```python
from build123d import *

# Parameters (mm, degrees)
SKETCH_1_W           = 76.35
SKETCH_1_H           = 54
EXTRUDE_7_DEPTH      = 5
EXTRUDE_7_DEPTH_BACK = 5
EXTRUDE_8_DEPTH      = 12.5
EXTRUDE_8_DEPTH_BACK = 80
SKETCH_3_W           = 4.5
SKETCH_3_H           = 4
SKETCH_3_W_2         = 4
SKETCH_3_H_2         = 40.6
EXTRUDE_9_DEPTH      = 12.5
SKETCH_5_R           = 1.25
CUT_EXTRUDE_1_DEPTH  = 12.5
FILLET_1_R           = 4
FILLET_2_R           = 4
FILLET_3_R           = 8
FILLET_4_R           = 8
FILLET_5_R           = 8
FILLET_6_R           = 8
FILLET_7_R           = 5
FILLET_8_R           = 5
FILLET_9_R           = 4
FILLET_10_R          = 4


with BuildPart() as part:
    # Sketch 1 → Extrude 7 (new body, two sides)
    with BuildSketch(Plane.XY) as extrude_7_sk:
        with Locations((38.175, -23)):
            Rectangle(SKETCH_1_W, SKETCH_1_H)
        Polygon((4, -46), (4, -39), (9, -39), (9, -36.6), (4, -36.6), (4, 0), (72.35, 0), (72.35, -36.6), (67.35, -36.6), (67.35, -39), (72.35, -39), (72.35, -46), align=None, mode=Mode.SUBTRACT)
    extrude(amount=EXTRUDE_7_DEPTH)
    extrude(extrude_7_sk.sketch, amount=-EXTRUDE_7_DEPTH_BACK)

    # Sketch 2 → Extrude 8 (add, two sides)
    with BuildSketch(Plane.XY.offset(5)) as extrude_8_sk:
        Polygon((4, -46), (4, -39), (9, -39), (9, -36.6), (4, -36.6), (0, -36.6), (0, -50), (76.35, -50), (76.35, -36.6), (72.35, -36.6), (67.35, -36.6), (67.35, -39), (72.35, -39), (72.35, -46), align=None)
    extrude(amount=EXTRUDE_8_DEPTH)
    extrude(extrude_8_sk.sketch, amount=-EXTRUDE_8_DEPTH_BACK)

    # Sketch 3 → Extrude 9 (add)
    with BuildSketch(Plane.XY.offset(5)):
        with Locations((52.065, 2)):
            Rectangle(SKETCH_3_W, SKETCH_3_H)
        with Locations((24.285, 2)):
            Rectangle(SKETCH_3_W, SKETCH_3_H)
        with Locations((2, -16.3)):
            Rectangle(SKETCH_3_W_2, SKETCH_3_H_2)
        with Locations((74.35, -16.3)):
            Rectangle(SKETCH_3_W_2, SKETCH_3_H_2)
    extrude(amount=EXTRUDE_9_DEPTH)

    # Sketch 5 → Cut-Extrude 1 (cut)
    with BuildSketch(Plane(origin=(0, 4, 0), x_dir=(1, 0, 0), z_dir=(0, 1, 0))):
        with Locations((24.285, -12.5)):
            Circle(SKETCH_5_R)
        with Locations((52.065, -12.5)):
            Circle(SKETCH_5_R)
    extrude(amount=-CUT_EXTRUDE_1_DEPTH, mode=Mode.SUBTRACT)

    # Fillet 1
    fillet_1_edges = [part.edges().sort_by_distance(p)[0] for p in [
        (2, -36.6, -5),
    ]]
    fillet(fillet_1_edges, radius=FILLET_1_R)

    # Fillet 2
    fillet_2_edges = [part.edges().sort_by_distance(p)[0] for p in [
        (74.35, -36.6, -5),
    ]]
    fillet(fillet_2_edges, radius=FILLET_2_R)

    # Fillet 3
    fillet_3_edges = [part.edges().sort_by_distance(p)[0] for p in [
        (4, 2, 5),
    ]]
    fillet(fillet_3_edges, radius=FILLET_3_R)

    # Fillet 4
    fillet_4_edges = [part.edges().sort_by_distance(p)[0] for p in [
        (72.35, 2, 5),
    ]]
    fillet(fillet_4_edges, radius=FILLET_4_R)

    # Fillet 5
    fillet_5_edges = [part.edges().sort_by_distance(p)[0] for p in [
        (22.035, 2, 5),
    ]]
    fillet(fillet_5_edges, radius=FILLET_5_R)

    # Fillet 6
    fillet_6_edges = [part.edges().sort_by_distance(p)[0] for p in [
        (54.315, 2, 5),
    ]]
    fillet(fillet_6_edges, radius=FILLET_6_R)

    # Fillet 7
    fillet_7_edges = [part.edges().sort_by_distance(p)[0] for p in [
        (72.35, 0, 0),
    ]]
    fillet(fillet_7_edges, radius=FILLET_7_R)

    # Fillet 8
    fillet_8_edges = [part.edges().sort_by_distance(p)[0] for p in [
        (4, 0, 0),
    ]]
    fillet(fillet_8_edges, radius=FILLET_8_R)

    # Fillet 9
    fillet_9_edges = [part.edges().sort_by_distance(p)[0] for p in [
        (4, -36.6, 6.25),
    ]]
    fillet(fillet_9_edges, radius=FILLET_9_R)

    # Fillet 10
    fillet_10_edges = [part.edges().sort_by_distance(p)[0] for p in [
        (72.35, -36.6, 6.25),
    ]]
    fillet(fillet_10_edges, radius=FILLET_10_R)


solid = part.part
```
Verification items for the finished model (mm, model axes). A direction names the side the tool comes from. Coordinates: 2 decimals unless noted, no trailing zeros. Loops run counter-clockwise (first coordinate to the right, second up) from the corner with the lowest first, then second, coordinate; pieces in that order, holes last. Notation, with made-up numbers: (20, -34) -> (70, -34) arc R10 ccw to (70, -19) -> close; hole circle Ø5 at (50.25, 45). An arc over 180 degrees is marked (long way). Put each result on its own line as item: value.
1. Gauge pin test, flat ends, axial feed: P1, Ø10, axis at x = 41, z = -26, coming from the +Y side; P2, Ø2.5, axis at x = 6, z = -42.5, coming from the +Y side; P3, Ø1.2, axis at x = 44, y = 2, coming from the +Z side; P4, Ø1, axis at y = -19.5, z = 4.5, coming from the -X side. Record the tip position at first contact, or that the pin passes through.
Result set:
P1: stops at y = -46
P2: stops at y = -36.6
P3: stops at z = 5
P4: stops at x = 0
2. Thickness scan on line 1 (X direction, y = 2.15, z = 12.5) (3 decimals); line 2 (X direction, y = -42.5, z = -31); line 3 (X direction, y = 1, z = 12) (3 decimals). Record the ranges inside material, lowest first.
Result set:
line 1: x = 0 to 4.016, 22.019 to 23.035, 25.535 to 26.535, 49.815 to 50.815, 53.315 to 54.331, 72.334 to 76.35
line 2: x = 0 to 4, 72.35 to 76.35
line 3: x = 0 to 4.063, 21.972 to 23.139, 25.431 to 26.535, 49.815 to 50.919, 53.211 to 54.378, 72.287 to 76.35
3. Section check C-C, the plane z = 0. Record the boundary of the cut face in (x, y), then the cut area to 3 significant figures.
Result set:
outline: (0, -50) -> (76.35, -50) -> (76.35, 4) -> (0, 4) -> close; hole (4, -46) -> (72.35, -46) -> (72.35, -39) -> (67.35, -39) -> (67.35, -36.6) -> (68.35, -36.6) arc R4 ccw to (72.35, -32.6) -> (72.35, -5) arc R5 ccw to (67.35, 0) -> (9, 0) arc R5 ccw to (4, -5) -> (4, -32.6) arc R4 ccw to (8, -36.6) -> (9, -36.6) -> (9, -39) -> (4, -39) -> close
area: 1,020 mm^2
4. Mould release check, pull along Y, two halves, no side actions. Record for faces 1 (the face through (38, 4, 1)), 2 (the face through (70, -39, -29)), 3 (the face through (37.6, -46.2, -75)), 4 (the face through (38, 0, 1)): pulls with the +Y half, pulls with the -Y half, needs draft (parallel to the pull), parting line crosses it, or undercut.
Result set:
face 1: pulls with the +Y half
face 2: undercut
face 3: needs draft
face 4: undercut
5. Section check D-D, the plane x = 34.5. Record the boundary of the cut face in (y, z).
Result set:
outline: (-50, -75) -> (-46, -75) -> (-46, 17.5) -> (-50, 17.5) -> close; (0, -5) -> (4, -5) -> (4, 5) -> (0, 5) -> close
6. Tool access check on faces 5 (the face through (5.4, 0.56, 8.48)), 6 (the face through (52.74, 2.03, 11.45)), 7 (the face through (70.92, -1.5, 1.87)), 8 (the face through (52, 2, 17.5)). Record the directions out of +Z, -Z, +X, -X, +Y, -Y that give a thin tool (end or side, any length) a straight path to the whole face; none if there is none.
Result set:
face 5: +Z, +Y
face 6: +Y
face 7: +Z, -Z
face 8: +Z, +X, -X, +Y, -Y
7. Section check B-B, the plane x = 6. Record the boundary of the cut face in (y, z).
Result set:
outline: (-50, -75) -> (-46, -75) -> (-46, 17.5) -> (-50, 17.5) -> close; (-39, -75) -> (-36.6, -75) -> (-36.6, -9) arc R4 cw to (-36.06, -7) -> (-36.06, 17.5) -> (-39, 17.5) -> close; (-1, -5) -> (4, -5) -> (4, 7.71) -> (-1, 7.71) -> close
8. Section check A-A, the plane y = -43.5. Record the boundary of the cut face in (x, z), then the cut area to 3 significant figures.
Result set:
outline: (0, -75) -> (4, -75) -> (4, 17.5) -> (0, 17.5) -> close; (72.35, -75) -> (76.35, -75) -> (76.35, 17.5) -> (72.35, 17.5) -> close
area: 740 mm^2
